Part model, mm, in its own coordinate system. Face numbers are marked on the shaded views. A direction names the side the tool comes from. Give positions to 0.01 mm unless a question says otherwise; leave off trailing zeros. Order: outer loops, then holes, each group sorted by start corner. A loop starts at its lowest first (then second) coordinate and runs counter-clockwise, first axis right, second up.
from build123d import *

# Parameters (mm, degrees)
SKETCH1_R               = 3.748314074
SKETCH1_R_2             = 2.15
BOSS_EXTRUDE1_DEPTH     = 1.1
BOSS_EXTRUDE2_START     = -2.5
BOSS_EXTRUDE2_DEPTH     = 5
SKETCH3_R               = 2.5
BOSS_EXTRUDE3_DEPTH     = 30.5
BOSS_EXTRUDE4_REACH     = 66.583
CUT_EXTRUDE1_DEPTH      = 77.014827373
CUT_EXTRUDE1_DEPTH_BACK = 77.014827373
SKETCH5_R               = 2.15
SKETCH6_R               = 1.15
BOSS_EXTRUDE5_DEPTH     = 2.5
SKETCH7_R               = 3
CUT_EXTRUDE2_DEPTH      = 1.3
BOSS_EXTRUDE6_START     = -7.5
SKETCH8_R               = 1.5
BOSS_EXTRUDE6_DEPTH     = 7.5
CUT_EXTRUDE3_DEPTH      = 77.681407452
CUT_EXTRUDE3_DEPTH_BACK = 77.681407452
SKETCH9_R               = 0.65


with BuildPart() as part:
    # Sketch1 → Boss-Extrude1 (new, symmetric)
    # profile 1 of 2: a face of its own
    with BuildSketch(Plane.XY):
        with BuildLine():
            Line((-29.007745084, 30.523910578), (-25.091893995, 35.069909945))
            ThreePointArc((-25.091893995, 35.069909945), (-29.621942143, 40.692126277), (-31.860472098, 47.55650071))
            Line((-31.860472098, 47.55650071), (-31.88258847, 47.720887837))
            ThreePointArc((-31.88258847, 47.720887837), (-31.857495615, 47.471553034), (-31.84911885, 47.221098797))
            ThreePointArc((-31.84911885, 47.221098797), (-34.80303687, 43.557931682), (-39.009027568, 45.6683978))
            Line((-39.009027568, 45.6683978), (-34.12097225, 34.928362615))
            Line((-34.12097225, 34.928362615), (-29.007745084, 30.523910578))
        make_face()
    # profile 2 of 2: a face of its own
    with BuildSketch(Plane.XY):
        with Locations((-35.597432924, 47.221098797)):
            Circle(SKETCH1_R)
        with Locations((-35.597432924, 47.221098797)):
            Circle(SKETCH1_R_2, mode=Mode.SUBTRACT)
    extrude(amount=BOSS_EXTRUDE1_DEPTH, both=True)

    # Boss-Extrude2: read off the stored shape, not the designer's step
    # Boss-Extrude2 outline → Boss-Extrude2 (add)
    with BuildSketch(Plane.XY.offset(BOSS_EXTRUDE2_START)):
        with BuildLine():
            ThreePointArc((-25.091893995, 35.069909945), (-26.003854199, 35.905963494), (-26.862376119, 36.796804144))
            ThreePointArc((-26.862376119, 36.796804144), (-27.511007835, 38.051535597), (-28.577777167, 38.977320299))
            ThreePointArc((-28.577777167, 38.977320299), (-29.726956647, 40.888456377), (-30.656228901, 42.915648441))
            Line((-30.656228901, 42.915648441), (-36.680056275, 40.551182055))
            Line((-36.680056275, 40.551182055), (-34.12097225, 34.928362615))
            ThreePointArc((-34.12097225, 34.928362615), (-32.905703874, 32.891668535), (-30.711472725, 31.991474297))
            Line((-30.711472725, 31.991474297), (-29.007745084, 30.523910578))
            Line((-29.007745084, 30.523910578), (-25.091893995, 35.069909945))
        make_face()
    extrude(amount=BOSS_EXTRUDE2_DEPTH)

    # Sketch3 → Boss-Extrude3 (add)
    with BuildSketch(Plane(origin=(-31.745759068, 27.345288728, 0), x_dir=(0, 0, -1), z_dir=(0.7576665611269928, -0.6526418482981281, 0))):
        with Locations((0, 7.195277993)):
            Circle(SKETCH3_R)
    extrude(amount=BOSS_EXTRUDE3_DEPTH)

    # Boss-Extrude4: up to this face of the body (flat: up to its plane)
    boss_extrude4_end = Plane(part.part.faces().sort_by_distance((-30.992912772, 36.816549457, 2.5))[0])
    # Sketch4 → Boss-Extrude4 (add, up to the picked face)
    with BuildSketch(Plane(origin=(0, 0, -2.5), x_dir=(-1, 0, 0), z_dir=(0, 0, -1)), mode=Mode.PRIVATE) as boss_extrude4_sk1:
        Polygon((44.67104718, 60.829350293), (38.62968166, 42.935799229), (36.680056275, 40.551182055), (34.487145344, 35.732918139), (39.271055483, 42.725492907), (45.31052994, 60.613442948), align=None)
    boss_extrude4_tool1 = split(extrude(boss_extrude4_sk1.sketch, amount=-BOSS_EXTRUDE4_REACH, mode=Mode.PRIVATE), bisect_by=boss_extrude4_end, keep=Keep.BOTH, mode=Mode.PRIVATE)
    add(boss_extrude4_tool1.solids().sort_by(Axis((-40.62976, 48.582602, -2.5), (0, 0, 1)))[0])

    # Sketch5 → Cut-Extrude1 (cut, two sides: drawn at the far end of the back side and taken through both)
    with BuildSketch(Plane.XY.offset(2.5).offset(-CUT_EXTRUDE1_DEPTH_BACK)):
        with Locations((-30.458296942, 35.732918139)):
            Circle(SKETCH5_R)
    extrude(amount=CUT_EXTRUDE1_DEPTH + CUT_EXTRUDE1_DEPTH_BACK, mode=Mode.SUBTRACT)

    # Sketch6 → Boss-Extrude5 (add, symmetric)
    with BuildSketch(Plane.XY):
        with BuildLine():
            Line((-3.018256327, 8.79690186), (-7.441885155, 12.607344927))
            Line((-7.441885155, 12.607344927), (-4.178675914, 16.395677733))
            Line((-4.178675914, 16.395677733), (1.686549766, 11.343466212))
            Line((1.686549766, 11.343466212), (1.686549766, 7.618415505))
            ThreePointArc((1.686549766, 7.618415505), (-1.420897666, 5.193336616), (-3.018256327, 8.79690186))
        make_face()
        with Locations((-0.813450234, 7.618415505)):
            Circle(SKETCH6_R, mode=Mode.SUBTRACT)
    extrude(amount=BOSS_EXTRUDE5_DEPTH, both=True)

    # Sketch7 → Cut-Extrude2 (cut, symmetric)
    with BuildSketch(Plane.XY):
        with Locations((-0.813450234, 7.618415505)):
            Circle(SKETCH7_R)
    extrude(amount=CUT_EXTRUDE2_DEPTH, both=True, mode=Mode.SUBTRACT)

    # Sketch8 → Boss-Extrude6 (add)
    with BuildSketch(Plane.XY.offset(2.5).offset(BOSS_EXTRUDE6_START)):
        with Locations(Location((-43.488619522, 59.906385053, 0), (0, 0, 255.286714902))):
            Circle(SKETCH8_R)
    extrude(amount=BOSS_EXTRUDE6_DEPTH)

    # Sketch9 → Cut-Extrude3 (cut, two sides: drawn at the far end of the back side and taken through both)
    with BuildSketch(Plane.XY.offset(2.5).offset(-CUT_EXTRUDE3_DEPTH_BACK)):
        with Locations((-43.488619522, 59.906385053)):
            Circle(SKETCH9_R)
    extrude(amount=CUT_EXTRUDE3_DEPTH + CUT_EXTRUDE3_DEPTH_BACK, mode=Mode.SUBTRACT)


with BuildPart() as part_1:
    # Body-Move/Copy1: moved
    add(part.part.moved(Location((35.6, -47.22, 0))))


with BuildPart() as body_2:
    # Split1: read off the stored shape, not the designer's step
    # Split1: the piece on the far side of the plane
    add(part_1.part)
    split(bisect_by=Plane.XY.offset(-2.5), keep=Keep.BOTTOM)


with BuildPart() as part_2:
    add(part_1.part)

    # Split1
    split(bisect_by=Plane.XY.offset(-2.5), keep=Keep.TOP)


with BuildPart() as body_2_1:
    # Body-Move/Copy2: read off the stored shape, not the designer's step
    # Body-Move/Copy2: moved
    add(body_2.part.moved(Location((0, 0, 7.5))))


with BuildPart() as part_3:
    add(part_2.part)

    # Combine1: read off the stored shape, not the designer's step
    # Combine1: union body 2
    add(body_2_1.part)


solid = part_3.part
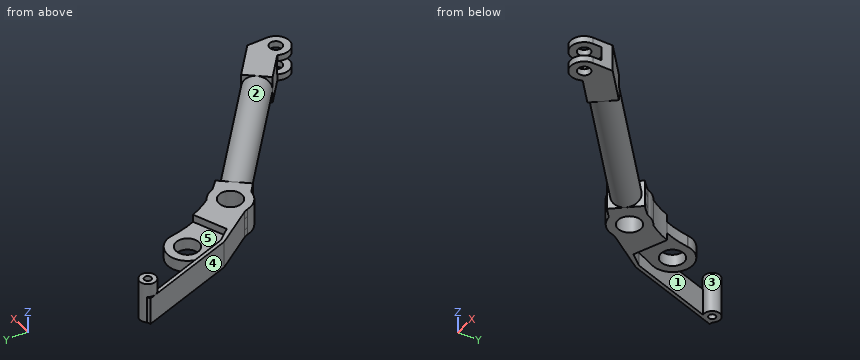
Item 1: Pull direction Y, two halves, no side cores. Call the marked faces 3, 4 and 5: released by +Y, released by -Y, zero draft, split by the parting line, or undercut.
Item 2: Drop flat-ended pins along their axis: P1, Ø8, axis at x = 9, y = -22, coming from the -Z side; P2, Ø3.5, axis at x = 0, y = 0, coming from the +Z side; P3, Ø7.5, axis at x = 31.5, y = -33.5, coming from the +Z side; P4, Ø10, axis at x = 4.5, y = 2.5, coming from the +Z side. Give the stop position or say it passes through.
Item 3: Band-saw the part on B-B on y = 10. List the corners of the cut face in (x, z).
Item 4: Which spindle directions (+Z, -Z, +X, -X, +Y, -Y) get a long thin tool onto all of the face, cutting with end or side? Do the marked faces 1 and 2. Say none if no direction does.
Item 5: Band-saw the part on A-A on z = 3.5. List the corners of the cut face in (x, y), plus the area to 3 significant figures.
Item 6: Drill centre lines: probe 1 along Y at (x, z) = (5, 0.5); probe 2 along Y at (x, z) = (35, 2); probe 3 along X at (y, z) = (-39, -1.75). Where is each one in solid material? Low to high.
Working result:
1. face 3: undercut
1. face 4: released by -Y
1. face 5: zero draft
2. P1: stops at z = -2.04
2. P2: passes through
2. P3: stops at z = 2.5
2. P4: stops at z = 1.1
3. outline: (-8.56, -2.5) - (-7.85, -2.5) - (-7.85, 2.5) - (-8.56, 2.5) - close
4. face 1: +Z, -Z
4. face 2: none
5. outline: circle Ø3 at (-7.89, 12.69); hole circle Ø1.3 at (-7.89, 12.69)
5. area: 5.74 mm2
6. probe 1: y = -15.32 to -13.63, -9.34 to -4.45
6. probe 2: y = -42.09 to -40.73, -38.47 to -33.91
6. probe 3: x = 32.36 to 33.81, 35.77 to 37.29
